Autodesk Inventor part; units mm, degrees
ref_plane "YZ Plane" through (0, 0, 0) normal (1, 0, 0) x (0, 1, 0)
ref_plane "XZ Plane" through (0, 0, 0) normal (0, 1, 0) x (-1, 0, 0)
ref_plane "XY Plane" through (0, 0, 0) normal (0, 0, 1) x (1, 0, 0)
sketch "Sketch1" plane through (0, 0, 0) normal (0, 1, 0) x (-1, 0, 0)
  line L0 (-10, -10) -> (10, -10)
  line L1 (10, -10) -> (10, 10)
  line L2 (10, 10) -> (-10, 10)
  line L3 (-10, 10) -> (-10, -10)
  line L4 (-10, -10) -> (10, 10) construction
  line L5 (10, -10) -> (-10, 10) construction
  point P0 (0, 0)
  dimension "d0" = 20
  dimension "d1" = 20
extrude "Extrusion1" add sketch "Sketch1" along normal blind 6.25
sketch "Sketch2" plane through (0, 6.25, 0) normal (0, 1, 0) x (1, 0, 0)
  line L0 (10, -7.5) -> (0, -7.5)
  line L1 (0, -7.5) -> (0, 7.5)
  line L2 (0, 7.5) -> (10, 7.5)
  line L3 (10, 7.5) -> (10, -7.5)
  line L4 (10, -10) -> (10, 10)
  line L5 (0, 0) -> (15, 0) construction
  line L6 (-15, 0) -> (20, 0) construction
  line L7 (-10, 10) -> (-10, -10) construction
  point P0 (0, 0)
  dimension "d4" = 15
  dimension "d5" = 10
extrude "Extrusion2" cut sketch "Sketch2" against normal blind 3
sketch "Sketch3" plane through (0, 3.25, 0) normal (0, 1, 0) x (1, 0, 0)
  line L0 (-14, 0) -> (14, 0) construction
  line L1 (10, -7.5) -> (0, -7.5) construction
  line L2 (10, -7.5) -> (0, -7.5) construction
  line L3 (5, -7.5) -> (5, 18.284) construction
  point P0 (0, 0)
  point P1 (5, -3.75)
  point P2 (5, 3.75)
  dimension "d8" = 7.5
  dimension "d26" = 3.75
hole "Hole1" at (5, 3.25, 3.75) at (5, 3.25, -3.75) direction (0, -1, 0) diameter 3 end through all
sketch "Sketch4" plane through (-10, 0, -10) normal (-1, 0, 0) x (0, 0, 1)
  line L0 (0, 0) -> (20, 0) construction
  line L1 (20, 0) -> (20, 6.25) construction
  line L2 (0, 6.25) -> (20, 6.25) construction
  line L3 (0, 0) -> (0, 6.25) construction
  line L4 (20, 3.125) -> (0, 3.125) construction
  line L5 (10, 0) -> (10, 6.25) construction
  point P0 (16, 3.125)
  point P1 (4, 3.125)
  dimension "d17" = 6
  dimension "d18" = 6
hole "Hole2" at (-10, 3.125, 6) at (-10, 3.125, -6) direction (1, 0, 0) diameter 2.459 depth 8.8 tip angle 118
fillet "Fillet1" radius 1.5 2 edges at (0, 4.75, -7.5) (0, 4.75, 7.5)
equation "\"d0\" = pillar_block_width"
equation "\"d1\" = pillar_block_length"
equation "\"d2\" = stock_6_width"
equation "\"d4\" = pillar_width"
equation "\"d6\" = stock_3_width"
equation "\"stock_6_width\" = 6.25"
equation "\"pillar_block_length\" = 20"
equation "\"pillar_block_width\" = 20"
equation "\"pillar_width\" = 15"
equation "\"stock_3_width\" = 3"
equation "\"pillar_length\" = 80"
properties part number "pillar_block" material "Aluminum 2014-T4"
Model file for the job. Use its own axes, mm. A direction names the side the tool comes from. Coordinates: 2 decimals unless noted, no trailing zeros. Loops run counter-clockwise (first coordinate to the right, second up) from the corner with the lowest first, then second, coordinate; pieces in that order, holes last. Notation, with made-up numbers: M 54.25,23 L 77.25,23 A11 cw 77.25,35 Z; hole C 65.25,-37 d5. An arc over 180 degrees is marked long. Use CSV: the item, a comma, the result in double quotes. Start each with the question number.
1. Band-saw the part on C-C, the plane y = 5.25. List the corners of the cut face in (x, z), then the cut area to 3 significant figures.
2. Band-saw the part on D-D, the plane z = 0.5. List the corners of the cut face in (x, y), then the cut area to 3 significant figures.
3. Probe probe 1 along Z at (x, y) = (-4.25, 3); probe 2 along Y at (x, z) = (-5, -6); probe 3 along X at (y, z) = (0.95, 3.75). List the from-to ranges inside material, lowest first. Write a range as [from, to].
4. Band-saw the part on A-A, the plane z = 3.75. List the corners of the cut face in (x, y).
5. Tool access for faces 4 (the flat face through (6, 5, -7.5)), 5 (the cylindrical face through (-5.54, 3.07, 4.77)), 6 (the cylindrical face through (4.55, 1.6, 5.18)): list every direction of +Z, -Z, +X, -X, +Y, -Y with a clear straight run to the whole face (end or side of a thin tool).
6. Band-saw the part on B-B, the plane x = 5. List the corners of the cut face in (y, z).
7. Two-plate mould, pull along Z, no slides. Class faces 1 (the flat face through (-2, 6.25, 0)), 2 (the flat face through (0, 3, 10)), 3 (the flat face through (5, 3.25, 0)): pulls with the +Z half, pulls with the -Z half, needs draft (parallel to the pull), parting line crosses it, or undercut.
8. Flat gauge pins, fed straight in: pin 1 (5 mm diameter, centred on x = 1, z = 1.5, fed in from -Y); pin 2 (4 mm diameter, centred on x = 4.5, z = 4.5, fed in from +Y). Where does each tip first touch, or does it go through?
Entries:
1,outline,"M -10,-10 L 10,-10 L 10,-7.5 L 1.5,-7.5 A1.5 cw 0,-6 L 0,6 A1.5 cw 1.5,7.5 L 10,7.5 L 10,10 L -10,10 Z"
1,area,"251 mm2"
2,outline,"M -10,0 L 10,0 L 10,3.25 L 0,3.25 L 0,6.25 L -10,6.25 Z"
2,area,"95.0 mm2"
3,probe 1,"z = [-10, -7.22], [-4.78, 4.78], [7.22, 10]"
3,probe 2,"y = [0, 1.9], [4.35, 6.25]"
3,probe 3,"x = [-10, 3.5], [6.5, 10]"
4,outline,"M -10,0 L 3.5,0 L 3.5,3.25 L 0,3.25 L 0,6.25 L -10,6.25 Z; M 6.5,0 L 10,0 L 10,3.25 L 6.5,3.25 Z"
5,face 4,"+X, +Y"
5,face 5,"-X"
5,face 6,"+Y, -Y"
6,outline,"M 0,-10 L 6.25,-10 L 6.25,-7.5 L 3.25,-7.5 L 3.25,-5.25 L 0,-5.25 Z; M 0,-2.25 L 3.25,-2.25 L 3.25,2.25 L 0,2.25 Z; M 0,5.25 L 3.25,5.25 L 3.25,7.5 L 6.25,7.5 L 6.25,10 L 0,10 Z"
7,face 1,"needs draft"
7,face 2,"pulls with the +Z half"
7,face 3,"undercut"
8,pin 1,"stops at y = 0"
8,pin 2,"stops at y = 3.25"
